```python
from build123d import *

# Parameters (mm, degrees)
SKETCH1_R           = 6.35
BOSS_EXTRUDE2_DEPTH = 7.62
CUT_EXTRUDE2_START  = -3.175
SKETCH3_R           = 6.35
CUT_EXTRUDE2_DEPTH  = 3.175
SKETCH4_W           = 25.4
SKETCH4_H           = 25.4
BOSS_EXTRUDE3_DEPTH = 50.8


with BuildPart() as part:
    # Sketch1 → Boss-Extrude2 (new body)
    with BuildSketch(Plane(origin=(0, 0, 0), x_dir=(1, 0, 0), z_dir=(0, 1, 0))):
        with BuildLine():
            Line((-76.2, 63.5), (76.2, 63.5))
            ThreePointArc((76.2, 63.5), (94.160512242, 56.060512242), (101.6, 38.1))
            Line((101.6, 38.1), (101.6, -38.1))
            ThreePointArc((101.6, -38.1), (94.160512242, -56.060512242), (76.2, -63.5))
            Line((76.2, -63.5), (-76.2, -63.5))
            ThreePointArc((-76.2, -63.5), (-94.160512242, -56.060512242), (-101.6, -38.1))
            Line((-101.6, -38.1), (-101.6, 38.1))
            ThreePointArc((-101.6, 38.1), (-94.160512242, 56.060512242), (-76.2, 63.5))
        make_face()
        with Locations(Location((-76.2, 38.1, 0), (0, 0, 90))):
            Circle(SKETCH1_R, mode=Mode.SUBTRACT)
        with Locations(Location((76.2, -38.1, 0), (0, 0, 90))):
            Circle(SKETCH1_R, mode=Mode.SUBTRACT)
        with Locations(Location((76.2, 38.1, 0), (0, 0, 90))):
            Circle(SKETCH1_R, mode=Mode.SUBTRACT)
        with Locations(Location((-76.2, -38.1, 0), (0, 0, 90))):
            Circle(SKETCH1_R, mode=Mode.SUBTRACT)
    extrude(amount=BOSS_EXTRUDE2_DEPTH)

    # Sketch3 → Cut-Extrude2 (cut)
    # profile 1 of 2: a face of its own
    with BuildSketch(Plane(origin=(0, 7.62, 0), x_dir=(1, 0, 0), z_dir=(0, 1, 0)).offset(CUT_EXTRUDE2_START)):
        with BuildLine():
            Line((-50.8, -63.5), (-50.8, 63.5))
            Line((-50.8, 63.5), (-76.2, 63.5))
            ThreePointArc((-76.2, 63.5), (-94.160512242, 56.060512242), (-101.6, 38.1))
            Line((-101.6, 38.1), (-101.6, -38.1))
            ThreePointArc((-101.6, -38.1), (-94.160512242, -56.060512242), (-76.2, -63.5))
            Line((-76.2, -63.5), (-50.8, -63.5))
        make_face()
        with Locations(Location((-76.2, -38.1, 0), (0, 0, 90))):
            Circle(SKETCH3_R, mode=Mode.SUBTRACT)
        with Locations(Location((-76.2, 38.1, 0), (0, 0, 90))):
            Circle(SKETCH3_R, mode=Mode.SUBTRACT)
    # profile 2 of 2: a face of its own
    with BuildSketch(Plane(origin=(0, 7.62, 0), x_dir=(1, 0, 0), z_dir=(0, 1, 0)).offset(CUT_EXTRUDE2_START)):
        with BuildLine():
            Line((76.2, 63.5), (50.8, 63.5))
            Line((50.8, 63.5), (50.8, -63.5))
            Line((50.8, -63.5), (76.2, -63.5))
            ThreePointArc((76.2, -63.5), (94.160512242, -56.060512242), (101.6, -38.1))
            Line((101.6, -38.1), (101.6, 38.1))
            ThreePointArc((101.6, 38.1), (94.160512242, 56.060512242), (76.2, 63.5))
        make_face()
        with Locations(Location((76.2, -38.1, 0), (0, 0, 90))):
            Circle(SKETCH3_R, mode=Mode.SUBTRACT)
        with Locations(Location((76.2, 38.1, 0), (0, 0, 90))):
            Circle(SKETCH3_R, mode=Mode.SUBTRACT)
    extrude(amount=CUT_EXTRUDE2_DEPTH, mode=Mode.SUBTRACT)

    # Sketch4 → Boss-Extrude3 (add)
    with BuildSketch(Plane.XZ):
        Rectangle(SKETCH4_W, SKETCH4_H)
    extrude(amount=BOSS_EXTRUDE3_DEPTH)


solid = part.part
```
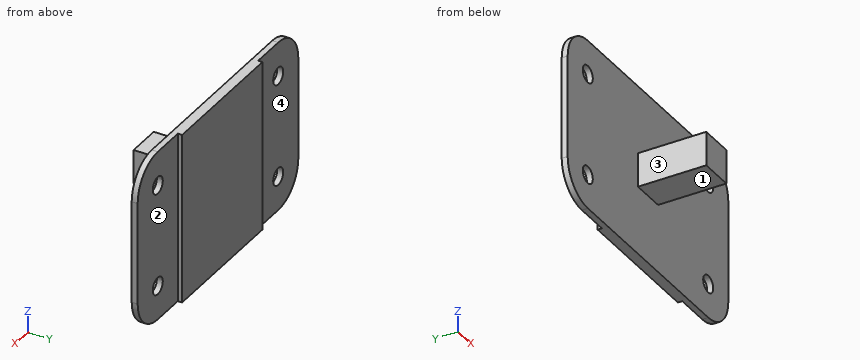
The listing builds one solid part. Answer for the finished solid, in the listing's coordinates (mm). Face numbers are marked on the shaded views. A direction names the side the tool comes from. Coordinates: 2 decimals unless noted, no trailing zeros. Loops run counter-clockwise (first coordinate to the right, second up) from the corner with the lowest first, then second, coordinate; pieces in that order, holes last. Notation, with made-up numbers: (-15.75, 8) -> (31.25, 8) arc R33 cw to (31.25, 43) -> close; hole circle Ø3 at (-30.5, -3.5). An arc over 180 degrees is marked (long way). Return JSON: item names as keys, results as strings. Group by question number.
(1) A cutting plane is placed at C-C on z = -42. Write down the section's boundary in (x, y) (3 decimals).
(2) Find the intervals of material crossed by probe 1 along Z at (x, y) = (-76, 1); probe 2 along X at (y, z) = (1.3, -38.1); probe 3 along Y at (x, z) = (3.5, -32.5), in increasing order. Write a range as from..to.
(3) A cutting plane is placed at A-A on z = 22.5. Write down the section's boundary in (x, y) (3 decimals).
(4) A cutting plane is placed at D-D on y = -25. Write down the section's boundary in (x, z), and give its area (3 significant figures).
(5) A cutting plane is placed at B-B on x = -6. Write down the section's boundary in (y, z).
(6) Which of the six approach directions +Z, -Z, +X, -X, +Y, -Y give full straight-line access (tool end or side, diameter ignored) to the marked faces 1, 2, 3 and 4?
(7) Given pin 1 Ø16.5 at (x, z) = (-76.2, 38.1) entering from +Y (3 decimals); pin 2 Ø20.5 at (x, y) = (-3.5, -13.5) entering from -Z; pin 3 Ø2.5 at (y, z) = (6, 27.5) entering from +X, each flat-ended and moving along its own axis, determine where each tip first touches the part or whether it passes through.
The answers:
{
 "1": {"outline": "(-101.299, 0) -> (-81.211, 0) -> (-81.211, 4.445) -> (-101.299, 4.445) -> close; (-71.189, 0) -> (71.189, 0) -> (71.189, 4.445) -> (50.8, 4.445) -> (50.8, 7.62) -> (-50.8, 7.62) -> (-50.8, 4.445) -> (-71.189, 4.445) -> close; (81.211, 0) -> (101.299, 0) -> (101.299, 4.445) -> (81.211, 4.445) -> close"},
 "2": {"probe 1": "z = -63.5..-44.45, -31.75..31.75, 44.45..63.5", "probe 2": "x = -101.6..-82.55, -69.85..69.85, 82.55..101.6", "probe 3": "y = 0..7.62"},
 "3": {"outline": "(-101.6, 0) -> (101.6, 0) -> (101.6, 4.445) -> (50.8, 4.445) -> (50.8, 7.62) -> (-50.8, 7.62) -> (-50.8, 4.445) -> (-101.6, 4.445) -> close"},
 "4": {"outline": "(-12.7, -12.7) -> (12.7, -12.7) -> (12.7, 12.7) -> (-12.7, 12.7) -> close", "area": "645 mm^2"},
 "5": {"outline": "(-50.8, -12.7) -> (0, -12.7) -> (0, -63.5) -> (7.62, -63.5) -> (7.62, 63.5) -> (0, 63.5) -> (0, 12.7) -> (-50.8, 12.7) -> close"},
 "6": {"face 1": "-Z, +X, -X, -Y", "face 2": "+Z, -Z, +X, +Y", "face 3": "+Z, -Z, -X, -Y", "face 4": "+Z, -Z, -X, +Y"},
 "7": {"pin 1": "stops at y = 4.445", "pin 2": "stops at z = -12.7", "pin 3": "stops at x = 50.8"}
}
